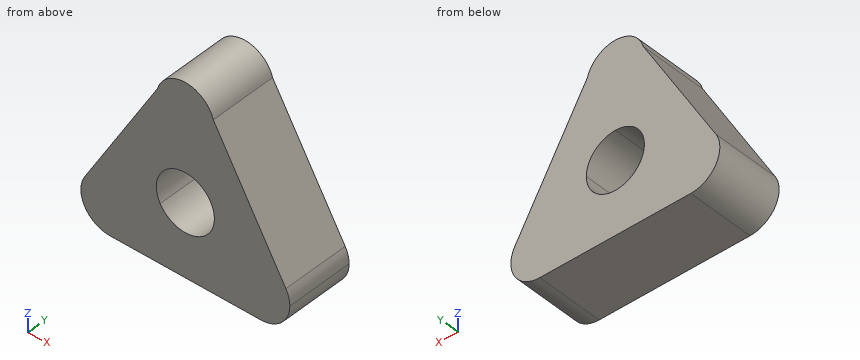
```python
from build123d import *

# Parameters (mm, degrees)
F1_DEPTH = 25.4


with BuildPart() as f1:
    # F0 (on Front) → F1 (new body)
    with BuildSketch(Plane.XZ):
        with BuildLine():
            ThreePointArc((0, 11), (7.778175, 7.778175), (11, 0))
            ThreePointArc((11, 0), (10.625184, -2.847009), (9.526279, -5.5))
            Line((9.526279, -5.5), (19.054118, -11.0009))
            ThreePointArc((19.054118, -11.0009), (28.544672, -5.501853), (38.069208, -10.941828))
            Line((38.069208, -10.941828), (10.584951, 35.986505))
            ThreePointArc((10.584951, 35.986505), (10.894398, 34.50748), (10.9982, 33))
            ThreePointArc((10.9982, 33), (7.776902, 25.223098), (0, 22.0018))
            Line((0, 22.0018), (0, 11))
        make_face()
        with BuildLine():
            ThreePointArc((-9.526279, -5.5), (-9.526279, 5.5), (0, 11))
            Line((0, 11), (0, 22.0018))
            ThreePointArc((0, 22.0018), (-8.769452, 26.362447), (-10.584951, 35.986505))
            Line((-10.584951, 35.986505), (-38.069208, -10.941828))
            ThreePointArc((-38.069208, -10.941828), (-28.544671, -5.501853), (-19.054118, -11.0009))
            Line((-19.054118, -11.0009), (-9.526279, -5.5))
        make_face()
        with BuildLine():
            Line((19.054118, -11.0009), (9.526279, -5.5))
            ThreePointArc((9.526279, -5.5), (0, -11), (-9.526279, -5.5))
            Line((-9.526279, -5.5), (-19.054118, -11.0009))
            ThreePointArc((-19.054118, -11.0009), (-17.955393, -13.653456), (-17.580638, -16.5))
            ThreePointArc((-17.580638, -16.5), (-20.801936, -24.276902), (-28.578838, -27.4982))
            Line((-28.578838, -27.4982), (28.578838, -27.4982))
            ThreePointArc((28.578838, -27.4982), (19.054118, -21.9991), (19.054118, -11.0009))
        make_face()
        with BuildLine():
            ThreePointArc((-10.584951, 35.986505), (-8.769452, 26.362447), (0, 22.0018))
            ThreePointArc((0, 22.0018), (7.776902, 25.223098), (10.9982, 33))
            ThreePointArc((10.9982, 33), (10.894398, 34.50748), (10.584951, 35.986505))
            ThreePointArc((10.584951, 35.986505), (0, 43.9982), (-10.584951, 35.986505))
        make_face()
        with BuildLine():
            ThreePointArc((38.069208, -10.941828), (28.544672, -5.501853), (19.054118, -11.0009))
            ThreePointArc((19.054118, -11.0009), (19.054118, -21.9991), (28.578838, -27.4982))
            ThreePointArc((28.578838, -27.4982), (36.35574, -24.276902), (39.577038, -16.5))
            ThreePointArc((39.577038, -16.5), (39.19339, -13.620467), (38.069208, -10.941828))
        make_face()
        with BuildLine():
            ThreePointArc((-17.580638, -16.5), (-17.955393, -13.653456), (-19.054118, -11.0009))
            ThreePointArc((-19.054118, -11.0009), (-28.544671, -5.501853), (-38.069208, -10.941828))
            ThreePointArc((-38.069208, -10.941828), (-38.120596, -21.969484), (-28.578838, -27.4982))
            ThreePointArc((-28.578838, -27.4982), (-20.801936, -24.276902), (-17.580638, -16.5))
        make_face()
    extrude(amount=F1_DEPTH)


solid = f1.part
```
CAD build for the part. Positions are in the model's coordinates, mm. Round coordinates to 2 decimals unless told otherwise and drop trailing zeros. Order: outer loops, then holes, each group sorted by start corner. A loop starts at its lowest first (then second) coordinate and runs counter-clockwise, first axis right, second up. Notation, with made-up numbers: (-27, 77) - (30, 77) arc R25 cw to (30, 109) - close; hole circle Ø11 at (-10, -16.75). An arc over 180 degrees is marked (long way). Use CSV: the item, a comma, the result in double quotes. Start each with the question number.
1) Saw through at D-D (z = 21.5). List the corners of the cut face in (x, y), and give its area (3 significant figures).
2) Saw through at C-C (y = -6.75). List the corners of the cut face in (x, z), and give its area (3 significant figures).
3) Saw through at B-B (z = 3). List the corners of the cut face in (x, y).
4) Pin check, flat tips, straight feed: pin 1 Ø10 at (y, z) = (-21, -7) entering from +X; pin 2 Ø4 at (x, z) = (23, -16.5) entering from +Y; pin 3 Ø3 at (y, z) = (-14.5, -4) entering from -X; pin 4 Ø4 at (x, z) = (29.5, 10) entering from -Y. Stop position of each tip, or through.
5) Wall check: L1, parallel to X at y = -6, z = 3.5; L2, parallel to X at y = -17, z = -9.5; L3, parallel to X at y = -18.5, z = 38.5. Give the ranges that are in metal, low to high. Write a range as [from, to].
6) Saw through at A-A (x = -4). List the corners of the cut face in (y, z).
Values follow:
1,outline,"(-19.07, -25.4) - (19.07, -25.4) - (19.07, 0) - (-19.07, 0) - close"
1,area,"969 mm2"
2,outline,"(-38.07, -10.94) arc R11 ccw to (-28.58, -27.5) - (28.58, -27.5) arc R11 ccw to (39.58, -16.5) arc R11 ccw to (38.07, -10.94) - (10.58, 35.99) arc R11 ccw to (-10.58, 35.99) - close; hole (0, 11) arc R11 ccw (long way) to (11, 0) arc R11 ccw to start"
2,area,"3,280 mm2"
3,outline,"(-29.9, -25.4) - (-10.58, -25.4) - (-10.58, 0) - (-29.9, 0) - close; (10.58, -25.4) - (29.9, -25.4) - (29.9, 0) - (10.58, 0) - close"
4,pin 1,"stops at x = 38.61"
4,pin 2,"stops at y = 0"
4,pin 3,"stops at x = -34.88"
4,pin 4,"passes through"
5,L1,"x = [-29.61, -10.43], [10.43, 29.61]"
5,L2,"x = [-37.22, -5.55], [5.55, 37.22]"
5,L3,"x = [-9.52, 9.52]"
6,outline,"(-25.4, -27.5) - (0, -27.5) - (0, -10.25) - (-25.4, -10.25) - close; (-25.4, 10.25) - (0, 10.25) - (0, 43.25) - (-25.4, 43.25) - close"
